For this review, take the finished solid that the model builds, in its own axes (mm). Coordinates: 2 decimals unless noted, no trailing zeros. Loops run counter-clockwise (first coordinate to the right, second up) from the corner with the lowest first, then second, coordinate; pieces in that order, holes last.
1. Take a section at C-C, the plane y = 1.4. Count the separate pieces of the cut face and the enclosed holes in it, then the cut area to 3 significant figures.
2. Mouldability with a two-part tool opening along Z and no side actions: class faces 1 (the face through (-27.53, 1.61, 123.98)), 2 (the face through (35, 3.175, -123)), 3 (the face through (120.94, 1.57, 92.73)) as pulls with the +Z half, pulls with the -Z half, needs draft (parallel to the pull), parting line crosses it, or undercut.
3. Take a section at B-B, the plane x = 102.5. State the section outline as (y, z) points (3 decimals), then the cut area to 3 significant figures.
4. To check wall thickness, follow probe 1 along Z at (x, y) = (0, 1.05); probe 2 along X at (y, z) = (0.7, -4); probe 3 along X at (y, z) = (1.3, -70). State the ranges of each line that lie inside material, in increasing order.
5. Clearance check with flat-ended pins moving along their axes: P1, Ø1, axis at y = 2, z = 19.5, coming from the -X side; P2, Ø5.5, axis at x = 119.11, z = 68.77, coming from the +Y side; P3, Ø1.5, axis at x = 60, y = 1.5, coming from the +Z side; P4, Ø1, axis at y = 2.5, z = -118.5, coming from the -X side. State where each tip first meets the part, or that it passes through.
6. Take a section at A-A, the plane z = 0. State the section outline as (x, y) points (3 decimals), then the cut area to 3 significant figures.
Autodesk Inventor part; units mm, degrees
ref_plane "YZ Plane" through (0, 0, 0) normal (1, 0, 0) x (0, 1, 0)
ref_plane "XZ Plane" through (0, 0, 0) normal (0, 1, 0) x (-1, 0, 0)
ref_plane "XY Plane" through (0, 0, 0) normal (0, 0, 1) x (1, 0, 0)
sketch "Sketch1" plane through (0, 0, 0) normal (0, 1, 0) x (-1, 0, 0)
  circle A0 centre (0, 0) radius 152.4
  dimension "d0" = 304.8
extrude "Extrusion1" add sketch "Sketch1" along normal blind 3.175
sketch "Sketch2" plane through (0, 3.175, 0) normal (0, 1, 0) x (1, 0, 0)
  circle A0 centre (0, 0) radius 137.541 construction
  circle A1 centre (0, -137.541) radius 3.175
  circle A2 centre (119.114, -68.7705) radius 3.175
  circle A3 centre (119.114, 68.7705) radius 3.175
  circle A4 centre (0, 137.541) radius 3.175
  circle A5 centre (-119.114, 68.7705) radius 3.175
  circle A6 centre (-119.114, -68.7705) radius 3.175
  dimension "d3" = 275.082
  dimension "d4" = 6.35
  dimension "d7" = 360
extrude "Extrusion2" cut sketch "Sketch2" against normal through all
sketch "Sketch3" plane through (0, 3.175, 0) normal (0, 1, 0) x (1, 0, 0)
  circle A0 centre (0, 0) radius 127
  dimension "d11" = 254
extrude "Extrusion3" cut sketch "Sketch3" against normal through all
sketch "Sketch5" plane through (0, 3.175, 0) normal (0, 1, 0) x (1, 0, 0)
  point P0 (0, 0)
  point P1 (0, 0)
properties part number "Top Plate"
Results list:
1. separate pieces: 1
1. enclosed holes: 7
1. area: 22,100 mm2
2. face 1: undercut
2. face 2: needs draft
2. face 3: parting line crosses it
3. outline: (0, -112.781) - (3.175, -112.781) - (3.175, -74.985) - (0, -74.985) - close; (0, 74.985) - (3.175, 74.985) - (3.175, 112.781) - (0, 112.781) - close
3. area: 240 mm2
4. probe 1: z = -152.4 to -140.72, -134.37 to -127, 127 to 134.37, 140.72 to 152.4
4. probe 2: x = -152.35 to -126.94, 126.94 to 152.35
4. probe 3: x = -135.37 to -122.04, -116.19 to -105.97, 105.97 to 116.19, 122.04 to 135.37
5. P1: stops at x = -151.21
5. P2: passes through
5. P3: stops at z = 140.41
5. P4: stops at x = -96.45
6. outline: (-152.4, 0) - (-127, 0) - (-127, 3.175) - (-152.4, 3.175) - close; (127, 0) - (152.4, 0) - (152.4, 3.175) - (127, 3.175) - close
6. area: 161 mm2
